Work out the finished part from the listing and answer in its coordinate system (mm). Coordinates: 2 decimals unless noted, no trailing zeros. Use a Markdown table: item, result. Add a question column.
(1) Find the intervals of material crossed by line 1 (X direction, y = 17, z = 3); line 2 (X direction, y = 16, z = 5.25); line 3 (Y direction, x = -11.5, z = 5.25), in increasing order. Write a range as from..to.
(2) For a pull along Y with two mould halves and no side action, classify faces 1 (the face through (45.46, 7.78, 3.03)), 2 (the face through (36.63, 21.73, 1.92)), 3 (the face through (0.698, 36.993, 2.972)) as released by +Y, released by -Y, zero draft, split by the parting line, or undercut.
(3) Given pin 1 Ø1 at (y, z) = (11.5, 1.5) entering from -X; pin 2 Ø2.5 at (x, y) = (-28, 31.31) entering from -Z; pin 3 Ø5.5 at (x, y) = (-12.53, 40.09) entering from -Z; pin 4 Ø1 at (y, z) = (37.5, 2.5) entering from +X, each flat-ended and moving along its own axis, determine where each tip first touches the part or whether it passes through.
from build123d import *

# Parameters (mm, degrees)
EXTRUDE_1_DEPTH           = 6
FILLET_1_R                = 3
HOLE_WIZARD_1_D           = 3.3
HOLE_WIZARD_1_DEPTH       = 7.5
HOLE_WIZARD_1_CSINK_D     = 7.5
HOLE_WIZARD_1_CSINK_ANGLE = 90
HOLE_WIZARD_1_TIP         = 0.991420021
FILLET_2_R                = 1


with BuildPart() as part:
    # 草图1 → 凸台-拉伸1 (new body)
    with BuildSketch(Plane.XY):
        with BuildLine():
            Line((-36.593586944, 5.468948212), (-46.483745578, 6.947042323))
            ThreePointArc((-46.483745578, 6.947042323), (0, 47), (46.483745578, 6.947042323))
            Line((46.483745578, 6.947042323), (36.593586944, 5.468948212))
            ThreePointArc((36.593586944, 5.468948212), (0, 37), (-36.593586944, 5.468948212))
        make_face()
    extrude(amount=EXTRUDE_1_DEPTH)

    # 圆角1
    fillet_1_edges = [part.edges().sort_by_distance(p)[0] for p in [
        (46.483745578, 6.947042323, 3),
        (36.593586944, 5.468948212, 3),
        (-36.593586944, 5.468948212, 3),
        (-46.483745578, 6.947042323, 3),
    ]]
    fillet(fillet_1_edges, radius=FILLET_1_R)

    # 打孔尺寸(%根据)内六角花形半沉头螺钉的类型1
    with Locations(Plane.XY.offset(6)):
        with Locations((-38.497337773, 16.790620208), (-27.999109004, 31.305656064), (-12.526872455, 40.088366806), (22.222162979, 35.639001962), (35.316348104, 22.730988481)):
            CounterSinkHole(HOLE_WIZARD_1_D / 2, HOLE_WIZARD_1_CSINK_D / 2, depth=HOLE_WIZARD_1_DEPTH, counter_sink_angle=HOLE_WIZARD_1_CSINK_ANGLE)
            with Locations((0, 0, -(HOLE_WIZARD_1_DEPTH + HOLE_WIZARD_1_TIP / 2))):  # 118° drill point
                Cone(0, HOLE_WIZARD_1_D / 2, HOLE_WIZARD_1_TIP, mode=Mode.SUBTRACT)

    # 圆角2
    fillet_2_edges = [part.edges().sort_by_distance(p)[0] for p in [
        (41.432322076, 6.192102022, 0),
        (41.432322076, 6.192102022, 6),
        (0, 47, 0),
        (0, 37, 0),
        (-41.432322076, 6.192102022, 0),
        (-37.313071306, 6.385935339, 0),
        (-45.443039337, 7.754357798, 0),
        (45.443039337, 7.754357798, 0),
        (37.313071306, 6.385935339, 0),
        (0, 37, 6),
        (0, 47, 6),
        (-41.432322076, 6.192102022, 6),
        (-37.313071306, 6.385935339, 6),
        (-45.443039337, 7.754357798, 6),
        (45.443039337, 7.754357798, 6),
        (37.313071306, 6.385935339, 6),
    ]]
    fillet(fillet_2_edges, radius=FILLET_2_R)


solid = part.part
Model answer:
| question | item | result |
|---|---|---|
| 1 | line 1 | -43.82..-40.13, -36.86..-32.86, 32.86..43.82 |
| 1 | line 2 | -44.16..-41.39, -35.6..-33.4, 33.4..44.16 |
| 1 | line 3 | 35.2..37.27, 42.91..45.54 |
| 2 | face 1 | split by the parting line |
| 2 | face 2 | undercut |
| 2 | face 3 | released by -Y |
| 3 | pin 1 | x = -45.69 |
| 3 | pin 2 | through |
| 3 | pin 3 | z = 0 |
| 3 | pin 4 | x = 28.98 |
